Autodesk Inventor part; units mm, degrees
ref_plane "YZ Plane" through (0, 0, 0) normal (1, 0, 0) x (0, 1, 0)
ref_plane "XZ Plane" through (0, 0, 0) normal (0, 1, 0) x (-1, 0, 0)
ref_plane "XY Plane" through (0, 0, 0) normal (0, 0, 1) x (1, 0, 0)
sketch "Sketch1" plane through (0, 0, 0) normal (0, 1, 0) x (-1, 0, 0)
  line L0 (50.8, 46.2915) -> (-50.8, 46.2915)
  line L1 (-50.8, 46.2915) -> (-50.8, -46.2915)
  line L2 (-50.8, -46.2915) -> (50.8, -46.2915)
  line L3 (50.8, -46.2915) -> (50.8, 46.2915)
  line L4 (50.8, 46.2915) -> (-50.8, -46.2915) construction
  line L5 (-50.8, 46.2915) -> (50.8, -46.2915) construction
  point P0 (0, 0)
  dimension "width" = 101.6
  dimension "depth" = 92.583
extrude "Extrusion1" add sketch "Sketch1" along normal blind 9.525
sketch "Sketch2" plane through (0, 9.525, 0) normal (0, 1, 0) x (1, 0, 0)
  line L0 (-12.7, -38.6715) -> (12.7, -38.6715) construction
  line L1 (12.7, -38.6715) -> (12.7, -13.2715) construction
  line L2 (12.7, -13.2715) -> (-12.7, -13.2715) construction
  line L3 (-12.7, -13.2715) -> (-12.7, -38.6715) construction
  line L4 (-12.7, -38.6715) -> (12.7, -13.2715) construction
  line L5 (12.7, -38.6715) -> (-12.7, -13.2715) construction
  line L6 (-50.8, -46.2915) -> (50.8, -46.2915)
  point P0 (0, 0)
  point P1 (0, -25.9715)
  dimension "d4" = 25.4
  dimension "d5" = 25.4
  dimension "d6" = 7.62
hole "Hole1" at (-12.7, 9.525, 38.6715) at (12.7, 9.525, 38.6715) at (12.7, 9.525, 13.2715) at (-12.7, 9.525, 13.2715) direction (0, -1, 0) diameter 5.1054 end through all counterbore diameter 8.128 counterbore depth 4.826
sketch "Sketch3" plane through (0, 9.525, 0) normal (0, 1, 0) x (1, 0, 0)
  line L0 (-50.8, 46.2915) -> (-50.8, -46.2915)
  line L1 (50.8, -46.2915) -> (50.8, 46.2915)
  line L2 (-50.8, -30.4165) -> (50.8, -30.4165)
  line L3 (50.8, -30.4165) -> (50.8, -20.8915)
  line L4 (50.8, -20.8915) -> (-50.8, -20.8915)
  line L5 (-50.8, -20.8915) -> (-50.8, -30.4165)
  line L6 (-50.8, -46.2915) -> (50.8, -46.2915)
  point P0 (0, 0)
  point P1 (-50.8, -20.8915)
  point P2 (50.8, -30.4165)
  dimension "d14" = 9.525
  dimension "d16" = 25.4
extrude "Extrusion2" add sketch "Sketch3" along normal blind 50.8 contours L4 L1 L2 L0
sketch "Sketch5" plane through (50.8, 9.525, 20.8915) normal (0, 0, -1) x (-1, 0, 0)
  circle A0 centre (50.8, 38.5045) radius 4.7625
  circle A1 centre (50.8, 38.5045) radius 4.7625
  point P0 (50.8, -9.525)
extrude "Extrusion4" cut sketch "Sketch5" against normal through all
sketch "Sketch6" plane through (0, 9.525, 0) normal (0, 1, 0) x (1, 0, 0)
  line L0 (50.8, 46.2915) -> (-50.8, 46.2915)
  line L1 (50.8, -20.8915) -> (50.8, 46.2915)
  line L2 (-50.8, 46.2915) -> (50.8, 46.2915)
  line L3 (50.8, 46.2915) -> (50.8, 36.7665)
  line L4 (50.8, 36.7665) -> (-50.8, 36.7665)
  line L5 (-50.8, 36.7665) -> (-50.8, 46.2915)
  point P0 (0, 0)
  dimension "d24" = 9.525
extrude "Extrusion5" add sketch "Sketch6" along normal blind 50.8
sketch "Sketch7" plane through (-50.8, 9.525, -36.7665) normal (0, 0, 1) x (1, 0, 0)
  circle A0 centre (50.8, 38.5045) radius 4.7625
  circle A1 centre (50.8, 38.5045) radius 4.7625
  point P0 (50.8, -9.525)
extrude "Extrusion6" cut sketch "Sketch7" against normal through all
sketch "Sketch8" plane through (0, 0, 0) normal (0, -1, 0) x (1, 0, 0)
  line L0 (-50.8, -46.2915) -> (-50.8, 46.2915)
  line L1 (50.8, -46.2915) -> (-50.8, -46.2915)
  line L2 (-50.8, 46.2915) -> (-31.75, 46.2915)
  line L3 (-31.75, 46.2915) -> (-31.75, -46.2915)
  line L4 (-31.75, -46.2915) -> (-50.8, -46.2915)
  line L5 (-50.8, -46.2915) -> (-50.8, 46.2915)
  line L6 (50.8, 46.2915) -> (31.75, 46.2915)
  line L7 (31.75, 46.2915) -> (31.75, -46.2915)
  line L8 (31.75, -46.2915) -> (50.8, -46.2915)
  line L9 (50.8, -46.2915) -> (50.8, 46.2915)
  point P0 (0, 0)
  dimension "d29" = 19.05
  dimension "d30" = 19.05
extrude "Extrusion7" cut sketch "Sketch8" against normal through all
sketch "Sketch9" plane through (0, 9.525, 0) normal (0, 1, 0) x (1, 0, 0)
  line L0 (31.75, 36.7665) -> (31.75, 46.2915)
  line L1 (-31.75, -20.8915) -> (31.75, -20.8915)
  line L2 (31.75, 36.7665) -> (21.59, 36.7665)
  line L3 (21.59, 36.7665) -> (21.59, -20.8915)
  line L4 (21.59, -20.8915) -> (31.75, -20.8915)
  line L5 (31.75, -20.8915) -> (31.75, 36.7665)
  point P0 (0, 0)
  point P1 (31.75, -20.8915)
  dimension "d33" = 10.16
extrude "Extrusion8" add sketch "Sketch9" along normal blind 76.4032
sketch "Sketch10" plane through (31.75, 0, 46.2915) normal (1, 0, 0) x (0, 0, -1)
  line L0 (25.4, 85.9282) -> (83.058, 85.9282)
  circle A0 centre (63.627, 85.9282) radius 11.1125
  line L1 (25.4, 60.325) -> (25.4, 85.9282)
  point P0 (46.2915, 0)
  point P1 (74.7395, 85.9282)
  point P2 (52.5145, 85.9282)
  dimension "d36" = 38.227
  dimension "d39" = 22.225
extrude "Extrusion9" cut sketch "Sketch10" against normal through all contours L0 A0 picked at (65.7312, 79.4369)
sketch "Sketch11" plane through (0, 9.525, 0) normal (0, 1, 0) x (1, 0, 0)
  line L0 (-31.75, 36.7665) -> (-31.75, -20.8915)
  line L1 (-31.75, -20.8915) -> (21.59, -20.8915)
  line L2 (-31.75, 36.7665) -> (-21.59, 36.7665)
  line L3 (-21.59, 36.7665) -> (-21.59, -20.8915)
  line L4 (-21.59, -20.8915) -> (-31.75, -20.8915)
  line L5 (-31.75, -20.8915) -> (-31.75, 36.7665)
  point P0 (0, 0)
  dimension "d40" = 10.16
extrude "Extrusion10" add sketch "Sketch11" along normal blind 50.8
equation "\"width\" = overallWidth"
equation "\"depth\" = overallDepth"
equation "\"overallWidth\" = 101.6"
equation "\"gapBetweeenMotorAndBasePlate\" = 0.635"
properties part number "plateForPot" material "ABS Plastic"
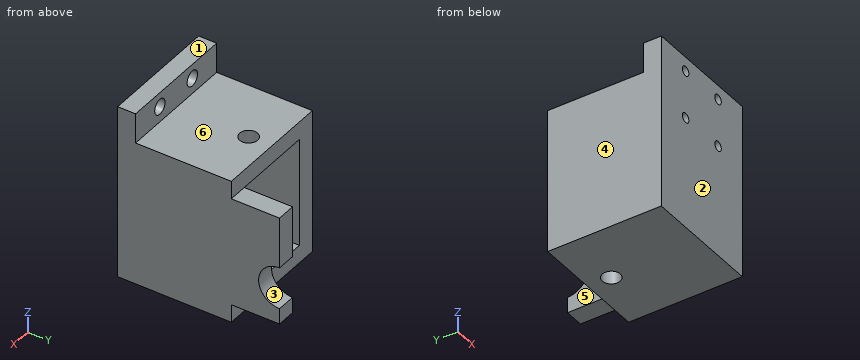
Verification items for the finished model (mm, model axes). Face numbers are marked on the shaded views. A direction names the side the tool comes from. Coordinates: 2 decimals unless noted, no trailing zeros. Write each loop counter-clockwise with the first axis right and the second up, starting at its lowest first coordinate (ties: lowest second). Pieces come first, ordered by that corner, then holes. Notation, with made-up numbers: (78.5, 49) -> (102.5, 49) arc R19 cw to (102.5, 73) -> close; hole circle Ø4 at (76.5, 13.5). An arc over 180 degrees is marked (long way). One line per item, written item: value. Start each with the question number.
Q1. Thickness scan on L1, parallel to Z at x = -12.7, y = 2.5; L2, parallel to X at y = 14, z = -33.5; L3, parallel to Z at x = 15, y = 54.5. Record the ranges inside material, lowest first. Write a range as from..to.
Q2. Mould release check, pull along Z, two halves, no side actions. Record for the marked faces 1, 2 and 3: pulls with the +Z half, pulls with the -Z half, needs draft (parallel to the pull), parting line crosses it, or undercut.
Q3. Cross-section at B-B on y = 42. Enter the section's corners in (x, z).
Q4. Cross-section at C-C on x = 12.7. Enter the section's corners in (y, z) (1 decimal).
Q5. Cross-section at A-A on x = 0. Enter the section's corners in (y, z) (1 decimal).
Q6. Go/stop test with flat-tipped pins: P1, Ø3, axis at x = 24.5, y = 67.5, coming from the -Z side; P2, Ø7.5, axis at x = -12.7, z = 38.67, coming from the +Y side; P3, Ø4, axis at x = 17, z = 29, coming from the +Y side (3 decimals). Record where each tip stops, or that it passes through.
Q7. Access from +Z, -Z, +X, -X, +Y, -Y to the whole of each face (thin tool, end or side, straight path). Record for the marked faces 4, 5 and 6.
Q8. Cross-section at D-D on y = 63. Enter the section's corners in (x, z).
Checked values:
1. L1: z = -46.29..10.72, 15.82..36.12, 41.22..46.29
1. L2: x = -31.75..-21.59, 21.59..31.75
1. L3: z = -46.29..-36.77, 20.89..30.42
2. face 1: pulls with the +Z half
2. face 2: needs draft
2. face 3: undercut
3. outline: (-31.75, -46.29) -> (31.75, -46.29) -> (31.75, 30.42) -> (-31.75, 30.42) -> close; hole (-21.59, -36.77) -> (21.59, -36.77) -> (21.59, 20.89) -> (-21.59, 20.89) -> close
4. outline: (0, -46.3) -> (60.3, -46.3) -> (60.3, -36.8) -> (9.5, -36.8) -> (9.5, 9.2) -> (4.7, 9.2) -> (4.7, 10.7) -> (0, 10.7) -> close; (0, 15.8) -> (4.7, 15.8) -> (4.7, 17.3) -> (9.5, 17.3) -> (9.5, 20.9) -> (60.3, 20.9) -> (60.3, 30.4) -> (9.5, 30.4) -> (9.5, 34.6) -> (4.7, 34.6) -> (4.7, 36.1) -> (0, 36.1) -> close; (0, 41.2) -> (4.7, 41.2) -> (4.7, 42.7) -> (9.5, 42.7) -> (9.5, 46.3) -> (0, 46.3) -> close
5. outline: (0, -46.3) -> (43.3, -46.3) -> (43.3, -36.8) -> (9.5, -36.8) -> (9.5, 20.9) -> (43.3, 20.9) -> (43.3, 30.4) -> (9.5, 30.4) -> (9.5, 46.3) -> (0, 46.3) -> close; (52.8, -46.3) -> (60.3, -46.3) -> (60.3, -36.8) -> (52.8, -36.8) -> close; (52.8, 20.9) -> (60.3, 20.9) -> (60.3, 30.4) -> (52.8, 30.4) -> close
6. P1: stops at z = -36.77
6. P2: stops at y = 4.7
6. P3: stops at y = 60.325
7. face 4: +Z, -Z, -X, +Y, -Y
7. face 5: +Y
7. face 6: +Z, +X, -X, +Y
8. outline: (21.59, -36.77) -> (31.75, -36.77) -> (31.75, 20.89) -> (21.59, 20.89) -> close
